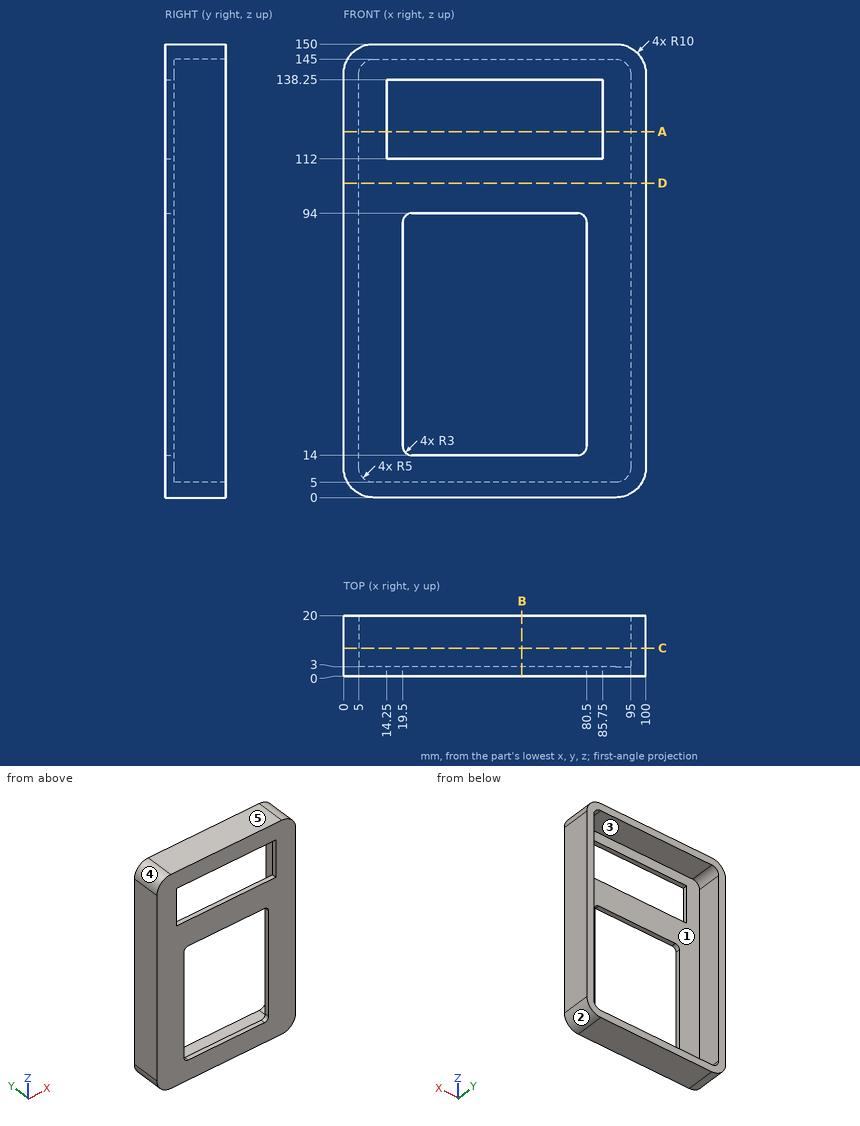
Job drawing, mm, ordinate dimensions from the low corner. One solid piece. A direction names the side the tool comes from. Coordinates: 2 decimals unless noted, no trailing zeros. Write each loop counter-clockwise with the first axis right and the second up, starting at its lowest first coordinate (ties: lowest second). Pieces come first, ordered by that corner, then holes. Notation, with made-up numbers: M 72,34 L 110,34 A12 ccw 110,44 Z; hole C 75,88.5 d11. An arc over 180 degrees is marked long. Answer as a JSON object with one key per item and string values. Group by question number.
1) Saw through at A-A (z = 121). Write the cut outline in (x, y), plus the area to 4 significant figures.
2) Saw through at B-B (x = 59). Write the cut outline in (y, z), plus the area to 3 significant figures.
3) Tool access for the marked faces 1 and 2: list every direction of +Z, -Z, +X, -X, +Y, -Y with a clear straight run to the whole face (end or side of a thin tool).
4) Wall check: line 1 (Z direction, x = 40, y = 1.25); line 2 (X direction, y = 8.5, z = 56); line 3 (Z direction, x = 68, y = 17.25). Give the ranges that are in metal, low to high. Write a range as from..to.
5) Mould opens along X. For the marked faces 3, 4 and 5 say: +X half, -X half, draft (parallel to the pull), parting line (faces both ways), or undercut.
6) Saw through at C-C (y = 9.25). Write the cut outline in (x, z), plus the area to 3 significant figures.
7) Saw through at D-D (z = 104). Write the cut outline in (x, y), plus the area to 3 significant figures.
Values follow:
{
 "1": {"outline": "M 0,0 L 14.25,0 L 14.25,3 L 5,3 L 5,20 L 0,20 Z; M 85.75,0 L 100,0 L 100,20 L 95,20 L 95,3 L 85.75,3 Z", "area": "255.5 mm2"},
 "2": {"outline": "M 0,0 L 20,0 L 20,5 L 3,5 L 3,14 L 0,14 Z; M 0,94 L 3,94 L 3,112 L 0,112 Z; M 0,138.25 L 3,138.25 L 3,145 L 20,145 L 20,150 L 0,150 Z", "area": "301 mm2"},
 "3": {"face 1": "+Y", "face 2": "-Z, +X, +Y, -Y"},
 "4": {"line 1": "z = 0..14, 94..112, 138.25..150", "line 2": "x = 0..5, 95..100", "line 3": "z = 0..5, 145..150"},
 "5": {"face 3": "undercut", "face 4": "-X half", "face 5": "draft"},
 "6": {"outline": "M 0,10 A10 ccw 10,0 L 90,0 A10 ccw 100,10 L 100,140 A10 ccw 90,150 L 10,150 A10 ccw 0,140 Z; hole M 5,10 A5 ccw 10,5 L 90,5 A5 ccw 95,10 L 95,140 A5 ccw 90,145 L 10,145 A5 ccw 5,140 Z", "area": "2,340 mm2"},
 "7": {"outline": "M 0,0 L 100,0 L 100,20 L 95,20 L 95,3 L 5,3 L 5,20 L 0,20 Z", "area": "470 mm2"}
}
